Design review of the part built by this model. Coordinates are the model's own, in mm. Coordinates: 2 decimals unless noted, no trailing zeros. Order: outer loops, then holes, each group sorted by start corner. A loop starts at its lowest first (then second) coordinate and runs counter-clockwise, first axis right, second up. Notation, with made-up numbers: (59, 63) -> (63, 63) arc R23 ccw to (63, 77) -> close; hole circle Ø7 at (77.25, 47.25). An arc over 180 degrees is marked (long way). Write item = value, one per line.
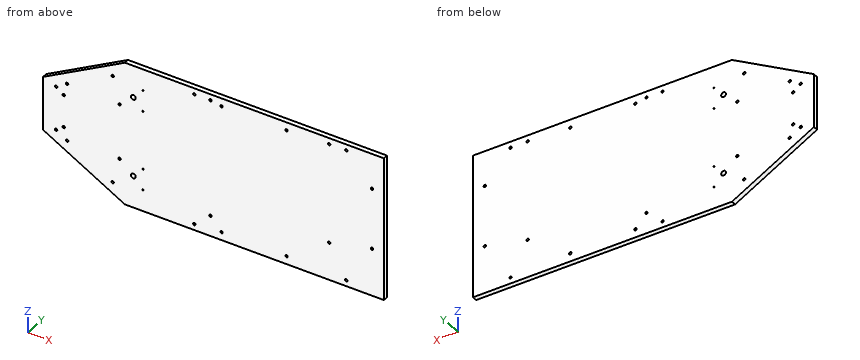
```python
from build123d import *

# Parameters (mm, degrees)
BOSS_EXTRUDE1_DEPTH = 6.35
SKETCH4_R           = 1.5875
SKETCH4_R_2         = 0.79502
SKETCH4_R_3         = 3.175
CUT_EXTRUDE1_DEPTH  = 7.35


with BuildPart() as part:
    # Sketch2 → Boss-Extrude1 (new body)
    with BuildSketch(Plane(origin=(0, 0, 0), x_dir=(1, 0, 0), z_dir=(0, 1, 0))):
        Polygon((-264.543396226, 98.724528302), (-264.543396226, 27.604528302), (-156.593396226, -32.085471698), (184.719103774, -32.085471698), (184.719103774, 158.414528302), (-156.593396226, 158.414528302), align=None)
    extrude(amount=BOSS_EXTRUDE1_DEPTH)

    # Sketch4 → Cut-Extrude1 (cut, through all)
    with BuildSketch(Plane(origin=(0, 6.35, 0), x_dir=(1, 0, 0), z_dir=(0, 1, 0))):
        with Locations((135.189103774, 150.413528302)):
            Circle(SKETCH4_R)
        with Locations((169.098103774, 14.650528302)):
            Circle(SKETCH4_R)
        with Locations((169.098103774, 95.422528302)):
            Circle(SKETCH4_R)
        with Locations((112.583103774, 108.376528302)):
            Circle(SKETCH4_R)
        with Locations((56.449103774, 147.619528302)):
            Circle(SKETCH4_R)
        with Locations((-29.275896226, 147.619528302)):
            Circle(SKETCH4_R)
        with Locations((-65.064496226, 150.413528302)):
            Circle(SKETCH4_R)
        with Locations((-43.880896226, 131.109528302)):
            Circle(SKETCH4_R)
        with Locations((-132.780896226, 129.839528302)):
            Circle(SKETCH4_R_2)
        with Locations((-132.780896226, 102.058278302)):
            Circle(SKETCH4_R_2)
        with Locations((-145.501812631, 115.948903302)):
            Circle(SKETCH4_R_3)
        with Locations((-237.238396226, 84.754528302)):
            Circle(SKETCH4_R)
        with Locations((-237.238396226, 41.759679404)):
            Circle(SKETCH4_R)
        with Locations((-163.578396226, 26.652028302)):
            Circle(SKETCH4_R)
        with Locations((-163.578396226, 99.677028302)):
            Circle(SKETCH4_R)
        with Locations((-247.271396226, 34.139679404)):
            Circle(SKETCH4_R)
        with Locations((-247.271396226, 92.1893772)):
            Circle(SKETCH4_R)
        with Locations((-232.793396226, 25.064528302)):
            Circle(SKETCH4_R)
        with Locations((-172.777199478, -8.120898136)):
            Circle(SKETCH4_R)
        with Locations((-172.777199478, 134.449954739)):
            Circle(SKETCH4_R)
        with Locations((-232.793396226, 101.264528302)):
            Circle(SKETCH4_R)
        with Locations((-132.780896226, -3.510471698)):
            Circle(SKETCH4_R_2)
        with Locations((-132.780896226, 24.270778302)):
            Circle(SKETCH4_R_2)
        with Locations((-145.501812631, 10.380153302)):
            Circle(SKETCH4_R_3)
        with Locations((-43.880896226, -24.084471698)):
            Circle(SKETCH4_R)
        with Locations((-29.275896226, -21.290471698)):
            Circle(SKETCH4_R)
        with Locations((56.449103774, -21.290471698)):
            Circle(SKETCH4_R)
        with Locations((135.189103774, -24.084471698)):
            Circle(SKETCH4_R)
        with Locations((112.583103774, -24.084471698)):
            Circle(SKETCH4_R)
        with Locations((-65.064496226, -24.084471698)):
            Circle(SKETCH4_R)
    extrude(amount=-CUT_EXTRUDE1_DEPTH, mode=Mode.SUBTRACT)


solid = part.part
```
(1) For L1, parallel to X at y = 3, z = -95.5; L2, parallel to Z at x = -162.5, y = 5.75; L3, parallel to Z at x = 111.5, y = 3, list the stretches that pass through material, from the lowest coordinate up.
Report:
L1 = -264.54 to 167.51, 170.68 to 184.72
L2 = -155.15 to -100.84, -98.51 to -27.82, -25.49 to 28.82
L3 = -158.41 to -109.54, -107.22 to 22.92, 25.25 to 32.09
(2) We need section B-B (x = -191.5). Write out the cut boundary in (y, z).
Report:
outline = (0, -139.11) -> (6.35, -139.11) -> (6.35, 12.78) -> (0, 12.78) -> close
(3) Insertion check: pin 1 (1.3 mm diameter, centred on x = -132.78, z = -24.27, fed in from +Y). The pin has a flat end and moves straight along its axis. Give the tip position at first contact, or say it passes through.
Report:
pin_1 = through
(4) We need section A-A (y = 4.5). Give the number of separate pieces and of enclosed holes in the cut face, and give its area (3 significant figures).
Report:
separate_pieces = 1
enclosed_holes = 30
area = 78,900 mm²
